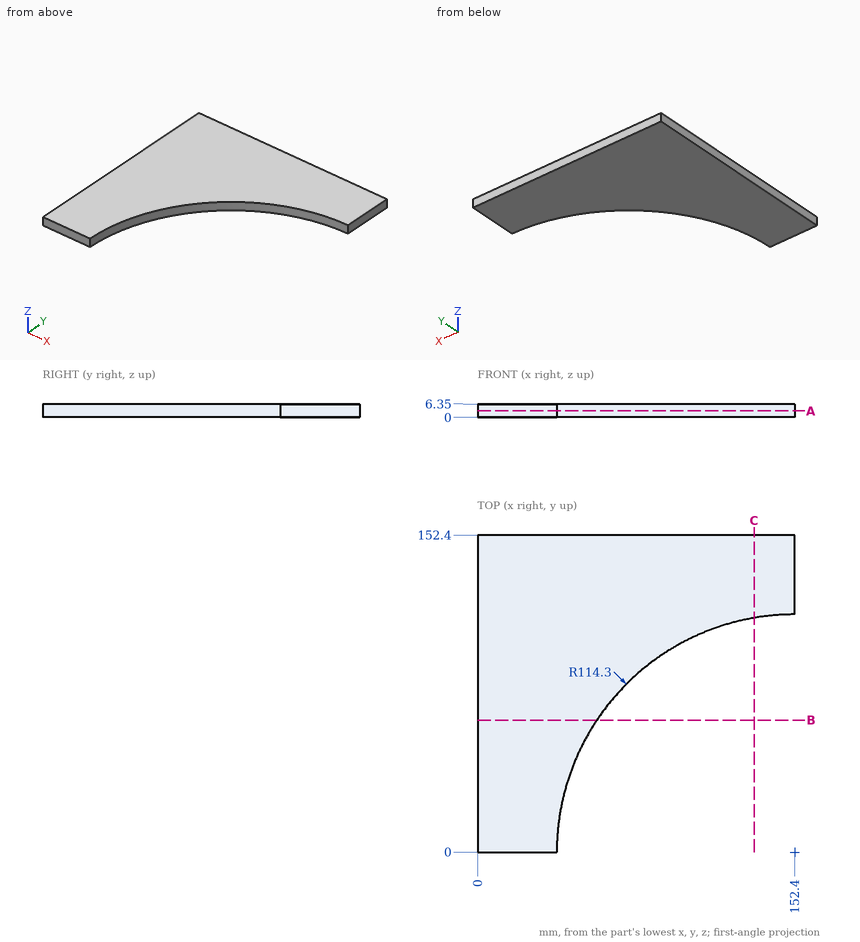
Could you check a few things on this drawing? It's one solid part, dimensions in mm from its lowest x, y, z. Round coordinates to 2 decimals unless told otherwise and drop trailing zeros. Order: outer loops, then holes, each group sorted by start corner. A loop starts at its lowest first (then second) coordinate and runs counter-clockwise, first axis right, second up. Notation, with made-up numbers: M 10.5,78.25 L 33.5,78.25 A13 cw 33.5,86.25 Z; hole C 1.5,73 d9. An arc over 180 degrees is marked long. One line per question, with ' | ' between items. Start each with the question number.
(1) Please list where these lines run through material, in increasing order: line 1 along X through (y, z) = (103, 1.25); line 2 along Y through (x, z) = (135.5, 5.25); line 3 along X through (y, z) = (14, 5.25).
(2) Suppose I cut it at B-B on y = 63.5. List the corners of the cut face in (x, z) for me.
(3) For P1, Ø1.5, axis at y = 59, z = 2.5, coming from the -X side; P2, Ø1.5, axis at x = 131.5, z = 4, coming from the -Y side; P3, Ø1.5, axis at y = 17, z = 1, coming from the +X side, each with a flat end and sliding along its axis, tell me the tip position at first contact or that it passes through.
(4) Suppose I cut it at A-A on z = 3. List the corners of the cut face in (x, y) for me.
(5) Suppose I cut it at C-C on x = 133. List the corners of the cut face in (y, z) for me.
Geometry results:
1) line 1: 0 to 102.85 | line 2: 113.04 to 152.4 | line 3: 0 to 38.96
2) outline: M 0,0 L 57.36,0 L 57.36,6.35 L 0,6.35 Z
3) P1: x = 0 | P2: y = 112.23 | P3: x = 39.49
4) outline: M 0,0 L 38.1,0 A114.3 cw 152.4,114.3 L 152.4,152.4 L 0,152.4 Z
5) outline: M 112.64,0 L 152.4,0 L 152.4,6.35 L 112.64,6.35 Z
